from build123d import *

# Parameters (mm, degrees)
F0_W     = 127
F0_H     = 50.8
F1_DEPTH = 38.1
F2_R     = 25.39999
F3_R     = 12.2082879552
F3_R_2   = 12.7
F4_DEPTH = 19.05
F5_R     = 12.7
F6_DEPTH = 50.8


# Not quite as in the source:
# - a fillet or chamfer is up to 0.001 mm smaller than in the source, because OpenCascade refuses the exact size


with BuildPart() as f1:
    # F0 (on Front) → F1 (new body)
    with BuildSketch(Plane.XZ):
        Rectangle(F0_W, F0_H)
    extrude(amount=F1_DEPTH)

    # F2 (radius 25.4 in the source; OpenCascade refuses exactly that, so slightly less here)
    f2_edges = [f1.edges().sort_by_distance(p)[0] for p in [
        (63.5, -19.05, 25.4),
        (63.5, -19.05, -25.4),
        (-63.5, -19.05, 25.4),
        (-63.5, -19.05, -25.4),
    ]]
    fillet(f2_edges, radius=F2_R)

    # F3 (on face) → F4 (cut)
    with BuildSketch(Plane(origin=(0, 0, 0), x_dir=(-1, 0, 0), z_dir=(0, 1, 0))):
        with Locations((47.625, 0)):
            Circle(F3_R)
        with Locations((-47.625, 0)):
            Circle(F3_R_2)
    extrude(amount=-F4_DEPTH, mode=Mode.SUBTRACT)

    # F5 (on face) → F6 (cut)
    with BuildSketch(Plane.XY.offset(25.4)):
        with Locations((0, -19.05)):
            Circle(F5_R)
    extrude(amount=-F6_DEPTH, mode=Mode.SUBTRACT)


solid = f1.part
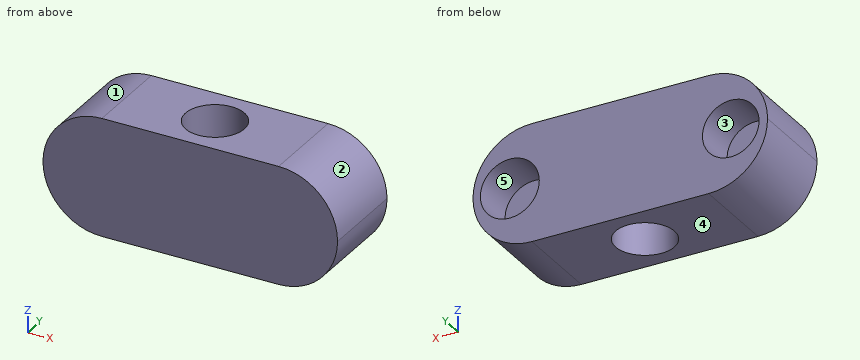
Could you check a few things on this model? Use its own coordinates, in mm. Face numbers are marked on the shaded views. A direction names the side the tool comes from. Give positions to 0.01 mm unless a question says otherwise; leave off trailing zeros. Order: outer loops, then holes, each group sorted by start corner. A loop starts at its lowest first (then second) coordinate and runs counter-clockwise, first axis right, second up.
Item 1: For the marked faces 4 and 5, which set-ups out of +Z, -Z, +X, -X, +Y, -Y let a thin tool reach every point of the face, with its end or its side?
Item 2: I'm going to push flat-ended pins straight in: pin 1 (14.5 mm diameter, centred on x = -47.625, z = 0, fed in from +Y); pin 2 (3 mm diameter, centred on y = -11.5, z = -13, fed in from -X); pin 3 (8 mm diameter, centred on x = -43, y = -29.5, fed in from -Z); pin 4 (20.5 mm diameter, centred on x = 0, y = -19.05, fed in from +Z). Where does each tip first touch, or does it pass through?
Item 3: If we section it at C-C, the plane z = -4.5: Write out the boundary of the cut face in (x, y).
Item 4: If we section it at B-B, the plane y = -3: Count the separate pieces of the cut face and the enclosed holes in it, plus the area to 3 significant figures.
Item 5: If we section it at A-A, the plane x = 0: Write out the boundary of the cut face in (y, z).
Item 6: I need wall thicknesses on line 1 (Y direction, x = 0, z = -6); line 2 (X direction, y = -13, z = 7); line 3 (Y direction, x = 47, z = -3.5). Which ranges of each line are inside material? Lowest first, please.
Item 7: If we mould it in two halves opening along X, with no side actions, what happens to the marked faces 1, 2 and 3? For each: pulls with the +X half, pulls with the -X half, needs draft (parallel to the pull), parting line crosses it, or undercut.
Values:
1. face 4: -Z, +X, -X, +Y, -Y
1. face 5: +Y
2. pin 1: stops at y = -19.05
2. pin 2: stops at x = -60.75
2. pin 3: stops at z = -25.38
2. pin 4: passes through
3. outline: (-63.1, -38.1) - (63.1, -38.1) - (63.1, 0) - (59.5, 0) - (59.5, -19.05) - (35.75, -19.05) - (35.75, 0) - (-36.28, 0) - (-36.28, -19.05) - (-58.97, -19.05) - (-58.97, 0) - (-63.1, 0) - close; hole circle Ø25.4 at (0, -19.05)
4. separate pieces: 1
4. enclosed holes: 2
4. area: 4,920 mm2
5. outline: (-38.1, -25.4) - (-31.75, -25.4) - (-31.75, 25.4) - (-38.1, 25.4) - close; (-6.35, -25.4) - (0, -25.4) - (0, 25.4) - (-6.35, 25.4) - close
6. line 1: y = -38.1 to -31.75, -6.35 to 0
6. line 2: x = -62.52 to -57.63, -37.62 to -11.17, 11.17 to 37.03, 58.22 to 62.52
6. line 3: y = -38.1 to -19.05
7. face 1: pulls with the -X half
7. face 2: pulls with the +X half
7. face 3: undercut
